```python
from build123d import *

# Parameters (mm, degrees)
F0_W      = 914.4
F0_H      = 152.4
F1_DEPTH  = 152.4
F2_W      = 127
F2_H      = 50.8
F3_DEPTH  = 101.6
F4_R      = 25.4
F5_DEPTH  = 337.82
F7_DEPTH  = 274.32
F9_DEPTH  = 492.76
F10_W     = 152.4
F10_H     = 38.1
F11_DEPTH = 63.5


with BuildPart() as f1:
    # F0 (on Front) → F1 (new body)
    with BuildSketch(Plane.XZ):
        Rectangle(F0_W, F0_H)
    extrude(amount=F1_DEPTH)

    # F2 (on face) → F3 (cut)
    with BuildSketch(Plane(origin=(0, 0, -76.2), x_dir=(1, 0, 0), z_dir=(0, 0, -1))):
        with Locations((-114.3, 76.2)):
            Rectangle(F2_W, F2_H)
    extrude(amount=-F3_DEPTH, mode=Mode.SUBTRACT)

    # F4 (on face) → F5 (cut)
    with BuildSketch(Plane.XZ.offset(152.4)):
        with Locations((-152.4, 25.4)):
            Circle(F4_R)
    extrude(amount=-F5_DEPTH, mode=Mode.SUBTRACT)

    # F6 (on face) → F7 (cut)
    with BuildSketch(Plane(origin=(0, 0, 0), x_dir=(-1, 0, 0), z_dir=(0, 1, 0))):
        with BuildLine():
            Line((130.4029547439, 38.1), (146.05, 38.1))
            Line((146.05, 38.1), (146.05, 49.9934442484))
            ThreePointArc((146.05, 49.9934442484), (137.0295007332, 45.6214676097), (130.4029547439, 38.1))
        make_face()
        with BuildLine():
            Line((-457.2, 38.1), (130.4029547439, 38.1))
            ThreePointArc((130.4029547439, 38.1), (137.0295007332, 45.6214676097), (146.05, 49.9934442484))
            Line((146.05, 49.9934442484), (146.05, 76.2))
            Line((146.05, 76.2), (-457.2, 76.2))
            Line((-457.2, 76.2), (-457.2, 38.1))
        make_face()
    extrude(amount=-F7_DEPTH, mode=Mode.SUBTRACT)

    # F8 (on face) → F9 (cut)
    with BuildSketch(Plane.YZ.offset(457.2)):
        with BuildLine():
            ThreePointArc((-88.9, 38.1), (-76.2, 25.4), (-63.5, 38.1))
            Line((-63.5, 38.1), (-88.9, 38.1))
        make_face()
    extrude(amount=-F9_DEPTH, mode=Mode.SUBTRACT)

    # F10 (on face) → F11 (cut)
    with BuildSketch(Plane.YZ.offset(457.2)):
        with Locations((-76.2, -19.05)):
            Rectangle(F10_W, F10_H)
    extrude(amount=-F11_DEPTH, mode=Mode.SUBTRACT)


solid = f1.part
```
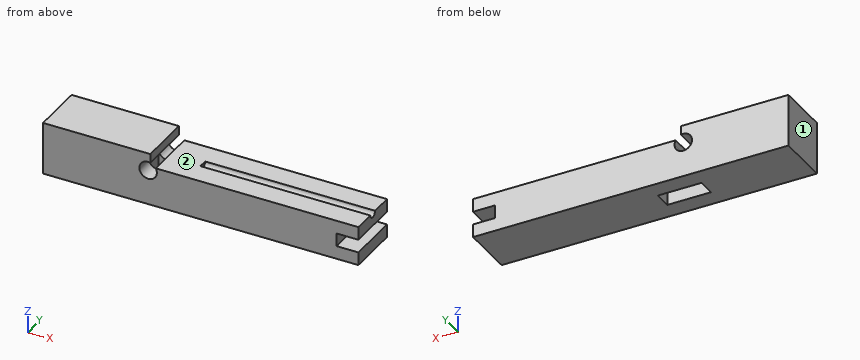
Part model, mm, in its own coordinate system. Face numbers are marked on the shaded views. A direction names the side the tool comes from. Round coordinates to 2 decimals unless told otherwise and drop trailing zeros. Write each loop counter-clockwise with the first axis right and the second up, starting at its lowest first coordinate (ties: lowest second). Pieces come first, ordered by that corner, then holes.
Item 1: Which spindle directions (+Z, -Z, +X, -X, +Y, -Y) get a long thin tool onto all of the face, cutting with end or side? Do the marked faces 1 and 2. Say none if no direction does.
Results:
face 1: +Z, -Z, -X, +Y, -Y
face 2: +Z, +X, +Y, -Y
Item 2: Drop flat-ended pins along their axis: pin 1 Ø2 at (x, y) = (116, -46.5) entering from +Z; pin 2 Ø10 at (y, z) = (-75.5, 30.5) entering from +X; pin 3 Ø1 at (x, y) = (15, -76.5) entering from +Z. Give the stop position or say it passes through.
Results:
pin 1: stops at z = 38.1
pin 2: stops at x = -35.56
pin 3: stops at z = 25.43
Item 3: Cut at D-D, the plane y = -127.5. Give the cut face in (x, z), plus the area to 3 significant figures.
Results:
outline: (-457.2, -76.2) - (457.2, -76.2) - (457.2, -38.1) - (393.7, -38.1) - (393.7, 0) - (457.2, 0) - (457.2, 38.1) - (-130.4, 38.1) arc R25.4 cw (long way) to (-146.05, 49.99) - (-146.05, 76.2) - (-457.2, 76.2) - close
area: 112,000 mm2
Item 4: Cut at B-B, the plane y = -76.2. Give the cut face in (x, z), plus the area to 3 significant figures.
Results:
outline: (-457.2, -76.2) - (-177.8, -76.2) - (-177.8, 25.4) arc R25.4 cw to (-146.05, 49.99) - (-146.05, 76.2) - (-457.2, 76.2) - close; (-130.4, 38.1) arc R25.4 cw to (-127, 25.4) - (-50.8, 25.4) - (-50.8, -76.2) - (457.2, -76.2) - (457.2, -38.1) - (393.7, -38.1) - (393.7, 0) - (457.2, 0) - (457.2, 25.4) - (-35.56, 25.4) - (-35.56, 38.1) - close
area: 93,900 mm2
Item 5: Cut at C-C, the plane x = 281.5. Give the cut face in (y, z), plus the area to 3 significant figures.
Results:
outline: (-152.4, -76.2) - (0, -76.2) - (0, 38.1) - (-63.5, 38.1) arc R12.7 cw to (-88.9, 38.1) - (-152.4, 38.1) - close
area: 17,200 mm2
Item 6: Cut at A-A, the plane z = -51.5. Give the cut face in (x, y), plus the area to 3 significant figures.
Results:
outline: (-457.2, -152.4) - (457.2, -152.4) - (457.2, 0) - (-457.2, 0) - close; hole (-177.8, -101.6) - (-50.8, -101.6) - (-50.8, -50.8) - (-177.8, -50.8) - close
area: 133,000 mm2
Item 7: Probe L1, parallel to X at y = -56.5, z = -61; L2, parallel to X at y = -79, z = -16; L3, parallel to Y at x = -118, z = 11.5. List the from-to ranges inside material, lowest first.
Results:
L1: x = -457.2 to -177.8, -50.8 to 457.2
L2: x = -457.2 to -177.8, -50.8 to 393.7
L3: y = -152.4 to -101.6, -50.8 to 0
